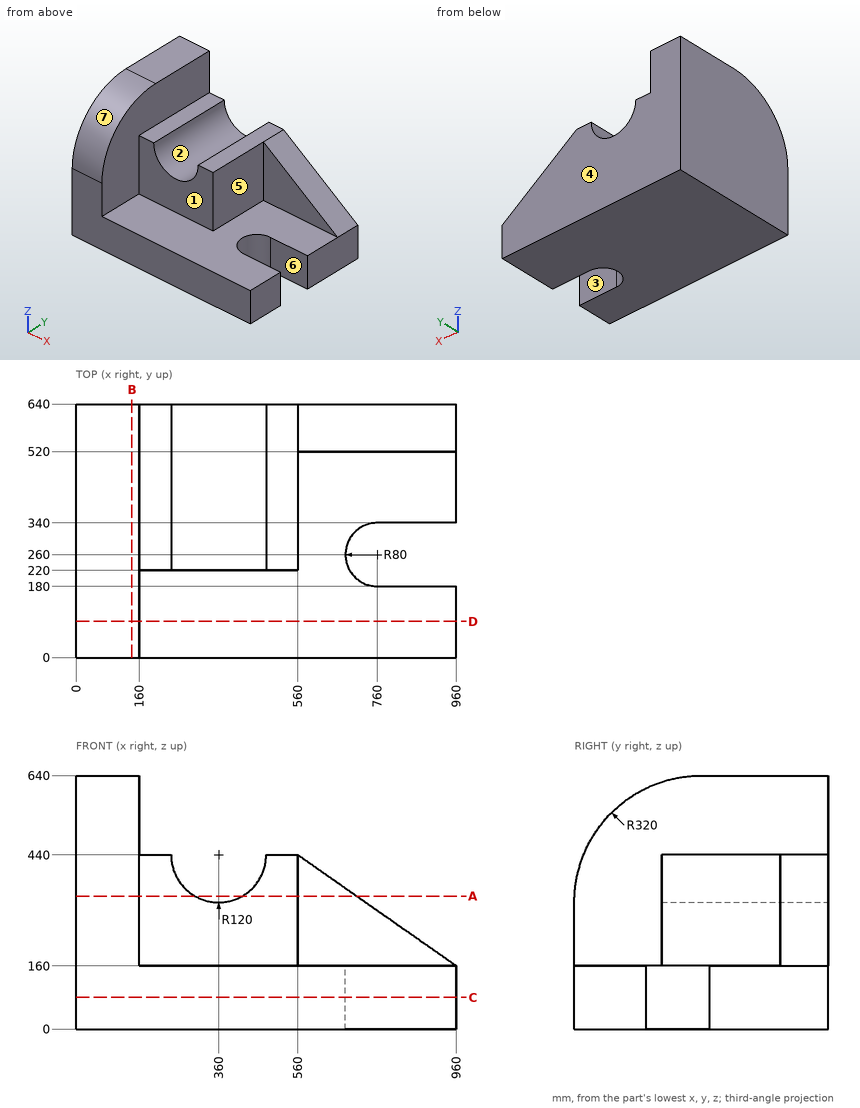
Geometry check sheet. Reference: drawing and pictorial views, mm from the part's lowest x, y, z. A direction names the side the tool comes from. Give positions to 0.01 mm unless a question says otherwise; leave off trailing zeros. Order: outer loops, then holes, each group sorted by start corner. A loop starts at its lowest first (then second) coordinate and runs counter-clockwise, first axis right, second up. Notation, with made-up numbers: M -4.75,70.5 L 54.25,70.5 A23 ccw 54.25,105.5 Z; hole C -35.75,63.25 d2. An arc over 180 degrees is marked long. Answer in a Markdown table with one row per item.
1) Release check for a two-part mould opening along Y. For the marked faces 4, 5, 6 and 7 record: +Y half, -Y half, draft (parallel to the pull), parting line (faces both ways), or undercut.
Filled sheet:
| item | result |
|---|---|
| face 4 | +Y half |
| face 5 | draft |
| face 6 | undercut |
| face 7 | -Y half |
2) Thickness scan on L1, parallel to Z at x = 558, y = 517; L2, parallel to X at y = 60, z = 321. Record the ranges inside material, lowest first. Write a range as [from, to].
Filled sheet:
| item | result |
|---|---|
| L1 | z = [0, 440] |
| L2 | x = [0, 160] |
3) Cross-section at D-D, the plane y = 91.5. Enter the section's corners in (x, z), plus the area to 3 significant figures.
Filled sheet:
| item | result |
|---|---|
| outline | M 0,0 L 960,0 L 960,160 L 160,160 L 160,544.03 L 0,544.03 Z |
| area | 215,000 mm2 |
4) Cross-section at A-A, the plane z = 336. Enter the section's corners in (x, y), plus the area to 3 significant figures.
Filled sheet:
| item | result |
|---|---|
| outline | M 0,0.4 L 160,0.4 L 160,220 L 300.13,220 L 300.13,640 L 0,640 Z; M 419.87,220 L 560,220 L 560,520 L 708.57,520 L 708.57,640 L 419.87,640 Z |
| area | 238,000 mm2 |
5) Cross-section at B-B, the plane x = 141. Enter the section's corners in (y, z), plus the area to 3 significant figures.
Filled sheet:
| item | result |
|---|---|
| outline | M 0,0 L 640,0 L 640,640 L 320,640 A320 ccw 0,320 Z |
| area | 388,000 mm2 |
6) Cross-section at C-C, the plane z = 80.5. Enter the section's corners in (x, y), plus the area to 3 significant figures.
Filled sheet:
| item | result |
|---|---|
| outline | M 0,0 L 960,0 L 960,180 L 760,180 A80 cw 760,340 L 960,340 L 960,640 L 0,640 Z |
| area | 572,000 mm2 |
7) Access from +Z, -Z, +X, -X, +Y, -Y to the whole of each face (thin tool, end or side, straight path). Record for the marked faces 1, 2 and 3.
Filled sheet:
| item | result |
|---|---|
| face 1 | +Z, +X, -Y |
| face 2 | +Z, +Y, -Y |
| face 3 | +Z, -Z, +X |
8) Gauge pin test, flat ends, axial feed: P1, Ø1, axis at x = 713, y = 382, coming from the +Z side; P2, Ø2, axis at x = 402.5, y = 270, coming from the +Z side; P3, Ø24, axis at x = 190.5, y = 398, coming from the +Z side. Record the tip position at first contact, or that the pin passes through.
Filled sheet:
| item | result |
|---|---|
| P1 | stops at z = 160 |
| P2 | stops at z = 328.16 |
| P3 | stops at z = 440 |
